Autodesk Inventor part; units mm, degrees
ref_plane "YZ Plane" through (0, 0, 0) normal (1, 0, 0) x (0, 1, 0)
ref_plane "XZ Plane" through (0, 0, 0) normal (0, 1, 0) x (-1, 0, 0)
ref_plane "XY Plane" through (0, 0, 0) normal (0, 0, 1) x (1, 0, 0)
sketch "Sketch1" plane through (0, 0, 0) normal (0, 0, 1) x (1, 0, 0)
  line L0 (-4.7625, -2.7496) -> (-4.7625, 2.7496)
  line L1 (-4.7625, 2.7496) -> (0, 5.4993)
  line L2 (0, 5.4993) -> (4.7625, 2.7496)
  line L3 (4.7625, 2.7496) -> (4.7625, -2.7496)
  line L4 (4.7625, -2.7496) -> (0, -5.4993)
  line L5 (0, -5.4993) -> (-4.7625, -2.7496)
  point P0 (0, 0)
  point P1 (0, 0)
  dimension "Size" = 9.525
extrude "Extrusion1" add sketch "Sketch1" along normal mid plane 73.025
sketch "Sketch3" plane through (0, 0, 36.5125) normal (0, 0, 1) x (1, 0, 0)
  line L0 (-4.7625, 2.7496) -> (0, 5.4993) construction
  line L1 (0, 5.4993) -> (4.7625, 2.7496) construction
  line L2 (4.7625, 2.7496) -> (4.7625, -2.7496) construction
  line L3 (4.7625, -2.7496) -> (0, -5.4993) construction
  line L4 (0, -5.4993) -> (-4.7625, -2.7496) construction
  line L5 (-4.7625, -2.7496) -> (-4.7625, 2.7496) construction
  point P0 (0, 0)
hole "Hole1" at (0, 0, 36.5125) direction (0, 0, -1) diameter 4.4958 end through all
sketch "Sketch4" plane through (0, 0, 36.5125) normal (0, 0, 1) x (1, 0, 0)
  circle A0 centre (0, 0) radius 2.2479 construction
  line L0 (-4.7625, 2.7496) -> (0, 5.4993) construction
  line L1 (0, 5.4993) -> (4.7625, 2.7496) construction
  line L2 (4.7625, 2.7496) -> (4.7625, -2.7496) construction
  line L3 (4.7625, -2.7496) -> (0, -5.4993) construction
  line L4 (0, -5.4993) -> (-4.7625, -2.7496) construction
  line L5 (-4.7625, -2.7496) -> (-4.7625, 2.7496) construction
  circle A1 centre (0, 0) radius 5.1245
  circle A2 centre (0, 0) radius 8.89
  dimension "thunder" = 10.2489
  dimension "d16" = 17.78
extrude "Extrusion3" cut sketch "Sketch4" against normal through all
equation "\"bearing\" = 25.4"
properties part number "GP1-004" material "Aluminum 6061"
Could you check a few things on this model? Use its own coordinates, in mm. Give positions to 0.01 mm unless a question says otherwise; leave off trailing zeros. Loops run counter-clockwise (first coordinate to the right, second up) from the corner with the lowest first, then second, coordinate; pieces in that order, holes last. Notation, with made-up numbers: M 43.5,50 L 76.5,50 A13 cw 76.5,68 Z; hole C 23,80 d1. An arc over 180 degrees is marked long. Answer as a JSON object with one key per item and string values.
Q1. For P1, Ø3.5, axis at x = 0, y = 0, coming from the +Z side; P2, Ø1.5, axis at x = -2, z = -23, coming from the +Y side; P3, Ø2, axis at y = -3, z = -22.5, coming from the +X side, each with a flat end and sliding along its axis, tell me the tip position at first contact or that it passes through.
Values found:
{"P1": "passes through", "P2": "stops at y = 4.78", "P3": "stops at x = 4.72"}
Q2. If I drill on probe 1 along Y at (x, z) = (-0.25, -2); probe 2 along X at (y, z) = (0, 7); probe 3 along Y at (x, z) = (2, -25.5), over which ranges is the centre line in solid material (lowest first)? Write a range as [from, to].
Values found:
{"probe 1": "y = [-5.12, -2.23], [2.23, 5.12]", "probe 2": "x = [-4.76, -2.25], [2.25, 4.76]", "probe 3": "y = [-4.34, -1.03], [1.03, 4.34]"}
Q3. Suppose I cut it at B-B, the plane y = 0. List the corners of the cut face in (x, z) for me.
Values found:
{"outline": "M -4.76,-36.51 L -2.25,-36.51 L -2.25,36.51 L -4.76,36.51 Z; M 2.25,-36.51 L 4.76,-36.51 L 4.76,36.51 L 2.25,36.51 Z"}
Q4. Suppose I cut it at C-C, the plane z = -28.5. List the corners of the cut face in (x, y) for me.
Values found:
{"outline": "M -4.76,-1.89 A5.12 ccw -4.02,-3.18 L -0.74,-5.07 A5.12 ccw 0.74,-5.07 L 4.02,-3.18 A5.12 ccw 4.76,-1.89 L 4.76,1.89 A5.12 ccw 4.02,3.18 L 0.74,5.07 A5.12 ccw -0.74,5.07 L -4.02,3.18 A5.12 ccw -4.76,1.89 Z; hole C 0,0 d4.5"}
Q5. Suppose I cut it at A-A, the plane x = 0. List the corners of the cut face in (y, z) for me, plus the area to 3 significant figures.
Values found:
{"outline": "M -5.12,-36.51 L -2.25,-36.51 L -2.25,36.51 L -5.12,36.51 Z; M 2.25,-36.51 L 5.12,-36.51 L 5.12,36.51 L 2.25,36.51 Z", "area": "420 mm²"}
Q6. Suppose I cut it at D-D, the plane x = 3. List the corners of the cut face in (y, z) for me, plus the area to 3 significant figures.
Values found:
{"outline": "M -3.77,-36.51 L 3.77,-36.51 L 3.77,36.51 L -3.77,36.51 Z", "area": "550 mm²"}
Q7. If we mould it in two halves opening along X, with no side actions, what happens to faces 1 (the cylindrical face through (4.443, 2.553, 0.511)), 2 (the flat face through (-2.2, 1.2, 36.512)), 3 (the flat face through (-2.404, 4.111, -0.511)), 4 (the cylindrical face through (0.861, -2.076, -0.511))? For each: pulls with the +X half, pulls with the -X half, needs draft (parallel to the pull), parting line crosses it, or undercut.
Values found:
{"face 1": "pulls with the +X half", "face 2": "needs draft", "face 3": "pulls with the -X half", "face 4": "undercut"}
